from build123d import *

# Parameters (mm, degrees)
BOSS_EXTRUDE1_DEPTH  = 0.762
BOSS_EXTRUDE2_DEPTH  = 2.54
SKETCH4_W            = 6.985
SKETCH4_H            = 4.572
BOSS_EXTRUDE3_DEPTH  = 1.27
FILLET1_R            = 2.54
SKETCH5_W            = 6.985
SKETCH5_H            = 2.032
BOSS_EXTRUDE4_DEPTH  = 0.508
FILLET2_R            = 1.016
FILLET3_R            = 1.016
FILLET2_OF_MIRROR4_R = 1.016
FILLET4_R            = 2.54
FILLET5_R            = 1.016


with BuildPart() as part:
    # Sketch1 → Boss-Extrude1 (new body)
    with BuildSketch(Plane.XY):
        Polygon((-33.378913043, 6.316869565), (16.151086957, 6.316869565), (24.088586957, -1.620630435), (16.151086957, -9.558130435), (-33.378913043, -9.558130435), (-41.316413043, -1.620630435), align=None)
    extrude(amount=BOSS_EXTRUDE1_DEPTH)

    # Sketch2 → Boss-Extrude2 (add)
    with BuildSketch(Plane(origin=(0, 0, 0), x_dir=(-1, 0, 0), z_dir=(0, 0, -1))):
        Polygon((30.521413043, 6.316869565), (33.378913043, 6.316869565), (41.316413043, -1.620630435), (33.378913043, -9.558130435), (30.521413043, -9.558130435), (30.521413043, -8.660104823), (32.480887431, -8.660104823), (39.520361819, -1.620630435), (32.480887431, 5.418843953), (30.521413043, 5.418843953), align=None)
        Polygon((-16.151086957, -9.558130435), (-24.088586957, -1.620630435), (-16.151086957, 6.316869565), (-13.293586957, 6.316869565), (-13.293586957, 5.418843953), (-15.253061344, 5.418843953), (-22.292535732, -1.620630435), (-15.253061344, -8.660104823), (-13.293586957, -8.660104823), (-13.293586957, -9.558130435), align=None)
    extrude(amount=BOSS_EXTRUDE2_DEPTH)

    # Sketch4 → Boss-Extrude3 (add)
    with BuildSketch(Plane(origin=(0, 6.316869565, 0), x_dir=(1, 0, 0), z_dir=(0, 1, 0))):
        with Locations((5.991086957, 1.524)):
            Rectangle(SKETCH4_W, SKETCH4_H)
        with Locations((-23.218913043, 1.524)):
            Rectangle(SKETCH4_W, SKETCH4_H)
    boss_extrude3 = extrude(amount=BOSS_EXTRUDE3_DEPTH)

    # Fillet1
    # the kernel refuses this fillet: 2.54 mm, written as the material it adds along each edge
    with BuildSketch(Plane(origin=(-26.711413043, 6.316869565, 0.762), x_dir=(-1, 0, 0), z_dir=(0, 0, -1)), Plane(origin=(-19.726413043, 6.316869565, 0), x_dir=(1, 0, 0), z_dir=(0, 0, 1)), Plane(origin=(2.498586957, 6.316869565, 0.762), x_dir=(-1, 0, 0), z_dir=(0, 0, -1)), Plane(origin=(9.483586957, 6.316869565, 0), x_dir=(1, 0, 0), z_dir=(0, 0, 1))) as fillet1_piece_1:
        with BuildLine():
            CenterArc((2.199704526, 2.54), FILLET1_R, 210, 60)
            Line((0, 1.27), (0, 0))
            Line((0, 0), (2.199704526, 0))
        make_face()
    extrude(amount=0.762)

    # Sketch5 → Boss-Extrude4 (add)
    with BuildSketch(Plane.XZ.offset(-6.316869565)):
        with Locations((5.991086957, -2.794)):
            Rectangle(SKETCH5_W, SKETCH5_H)
        with Locations((-23.218913043, -2.794)):
            Rectangle(SKETCH5_W, SKETCH5_H)
    boss_extrude4 = extrude(amount=BOSS_EXTRUDE4_DEPTH)

    # Fillet2
    # the kernel refuses this fillet: 1.016 mm, written as the material it takes off along each edge
    with BuildSketch(Plane(origin=(-0.041413043, 5.808869565, -3.81), x_dir=(0, 1, 0), z_dir=(1, 0, 0))) as fillet2_piece_1:
        with BuildLine():
            CenterArc((FILLET2_R, FILLET2_R), FILLET2_R, 180, 90)
            Line((0, FILLET2_R), (-FILLET2_R * 0.02, FILLET2_R))
            Line((-FILLET2_R * 0.02, FILLET2_R), (-FILLET2_R * 0.02, -FILLET2_R * 0.02))
            Line((-FILLET2_R * 0.02, -FILLET2_R * 0.02), (FILLET2_R, -FILLET2_R * 0.02))
            Line((FILLET2_R, -FILLET2_R * 0.02), (FILLET2_R, 0))
        make_face()
    extrude(amount=12.065, mode=Mode.SUBTRACT)
    with BuildSketch(Plane(origin=(11.683291482, 5.808869565, -1.778), x_dir=(0, 0, -1), z_dir=(-1, 0, 0))) as fillet2_piece_2:
        with BuildLine():
            CenterArc((0.87988181, -1.016), FILLET2_R, 90, 60)
            Line((0, -0.508), (-0.017597636, -0.49784))
            ThreePointArc((-0.017597636, -0.49784), (-0.02032, -0.254), (-0.02032, 0))
            Line((-0.02032, 0), (0, 0.02032))
            Line((0, 0.02032), (0.87988181, 0.02032))
            Line((0.87988181, 0.02032), (0.87988181, 0))
        make_face()
    extrude(amount=11.384409051, mode=Mode.SUBTRACT)
    with BuildSketch(Plane(origin=(-29.251413043, 5.808869565, -3.81), x_dir=(0, 0, 1), z_dir=(1, 0, 0))) as fillet2_piece_3:
        with BuildLine():
            CenterArc((FILLET2_R, -FILLET2_R), FILLET2_R, 90, 90)
            Line((0, -FILLET2_R), (-FILLET2_R * 0.02, -FILLET2_R))
            Line((-FILLET2_R * 0.02, -FILLET2_R), (-FILLET2_R * 0.02, FILLET2_R * 0.02))
            Line((-FILLET2_R * 0.02, FILLET2_R * 0.02), (FILLET2_R, FILLET2_R * 0.02))
            Line((FILLET2_R, FILLET2_R * 0.02), (FILLET2_R, 0))
        make_face()
    extrude(amount=12.065, mode=Mode.SUBTRACT)
    with BuildSketch(Plane(origin=(-17.526708518, 5.808869565, -1.778), x_dir=(0, 1, 0), z_dir=(-1, 0, 0))) as fillet2_piece_4:
        with BuildLine():
            CenterArc((1.016, 0.87988181), FILLET2_R, 180, 60)
            Line((0, 0.87988181), (-0.02032, 0.87988181))
            Line((-0.02032, 0.87988181), (-0.02032, 0))
            Line((-0.02032, 0), (0, -0.02032))
            ThreePointArc((0, -0.02032), (0.254, -0.02032), (0.49784, -0.017597636))
            Line((0.49784, -0.017597636), (0.508, 0))
        make_face()
    extrude(amount=11.384409051, mode=Mode.SUBTRACT)

    # Fillet3
    # the kernel refuses this fillet: 1.016 mm, written as the material it adds along each edge
    with BuildSketch(Plane(origin=(-26.711413043, 10.126869565, 0), x_dir=(-1, 0, 0), z_dir=(0, -1, 0))) as fillet3_piece_1_section:
        with BuildLine():
            CenterArc((FILLET3_R, FILLET3_R), FILLET3_R, 180, 90)
            Line((0, FILLET3_R), (0, 0))
            Line((0, 0), (FILLET3_R, 0))
        make_face()
    fillet3_piece_1 = extrude(amount=3.81, mode=Mode.PRIVATE)
    fillet3_piece_1 = fillet3_piece_1 - Plane(origin=(-28.911117569, 8.856869565, 0), x_dir=(-1, 0, 0), z_dir=(0, 0, 1)) * Cylinder(2.54, 12, mode=Mode.PRIVATE)
    add(fillet3_piece_1)
    with BuildSketch(Plane(origin=(-19.726413043, 10.126869565, 0), x_dir=(1, 0, 0), z_dir=(0, -1, 0))) as fillet3_piece_2_section:
        with BuildLine():
            CenterArc((FILLET3_R, -FILLET3_R), FILLET3_R, 90, 90)
            Line((0, -FILLET3_R), (0, 0))
            Line((0, 0), (FILLET3_R, 0))
        make_face()
    fillet3_piece_2 = extrude(amount=3.81, mode=Mode.PRIVATE)
    fillet3_piece_2 = fillet3_piece_2 - Plane(origin=(-17.526708518, 8.856869565, 0), x_dir=(1, 0, 0), z_dir=(0, 0, -1)) * Cylinder(2.54, 12, mode=Mode.PRIVATE)
    add(fillet3_piece_2)
    with BuildSketch(Plane(origin=(2.498586957, 10.126869565, 0), x_dir=(-1, 0, 0), z_dir=(0, -1, 0))) as fillet3_piece_3_section:
        with BuildLine():
            CenterArc((FILLET3_R, FILLET3_R), FILLET3_R, 180, 90)
            Line((0, FILLET3_R), (0, 0))
            Line((0, 0), (FILLET3_R, 0))
        make_face()
    fillet3_piece_3 = extrude(amount=3.81, mode=Mode.PRIVATE)
    fillet3_piece_3 = fillet3_piece_3 - Plane(origin=(0.298882431, 8.856869565, 0), x_dir=(-1, 0, 0), z_dir=(0, 0, 1)) * Cylinder(2.54, 12, mode=Mode.PRIVATE)
    add(fillet3_piece_3)
    with BuildSketch(Plane(origin=(9.483586957, 10.126869565, 0), x_dir=(1, 0, 0), z_dir=(0, -1, 0))) as fillet3_piece_4_section:
        with BuildLine():
            CenterArc((FILLET3_R, -FILLET3_R), FILLET3_R, 90, 90)
            Line((0, -FILLET3_R), (0, 0))
            Line((0, 0), (FILLET3_R, 0))
        make_face()
    fillet3_piece_4 = extrude(amount=3.81, mode=Mode.PRIVATE)
    fillet3_piece_4 = fillet3_piece_4 - Plane(origin=(11.683291482, 8.856869565, 0), x_dir=(1, 0, 0), z_dir=(0, 0, -1)) * Cylinder(2.54, 12, mode=Mode.PRIVATE)
    add(fillet3_piece_4)

    # Mirror4: Boss-Extrude3, Boss-Extrude4 across plane
    add(boss_extrude3.mirror(Plane.ZX.offset(-1.620630435)))
    add(boss_extrude4.mirror(Plane.ZX.offset(-1.620630435)))

    # Fillet2 of Mirror4
    # the kernel refuses this fillet: 1.016 mm, written as the material it takes off along each edge
    with BuildSketch(Plane(origin=(-0.041413043, -9.050130435, -3.81), x_dir=(0, 0, 1), z_dir=(1, 0, 0)), Plane(origin=(-29.251413043, -9.050130435, -3.81), x_dir=(0, 0, 1), z_dir=(1, 0, 0))) as fillet2_of_mirror4_piece_1:
        with BuildLine():
            CenterArc((FILLET2_OF_MIRROR4_R, FILLET2_OF_MIRROR4_R), FILLET2_OF_MIRROR4_R, 180, 90)
            Line((0, FILLET2_OF_MIRROR4_R), (-FILLET2_OF_MIRROR4_R * 0.02, FILLET2_OF_MIRROR4_R))
            Line((-FILLET2_OF_MIRROR4_R * 0.02, FILLET2_OF_MIRROR4_R), (-FILLET2_OF_MIRROR4_R * 0.02, -FILLET2_OF_MIRROR4_R * 0.02))
            Line((-FILLET2_OF_MIRROR4_R * 0.02, -FILLET2_OF_MIRROR4_R * 0.02), (FILLET2_OF_MIRROR4_R, -FILLET2_OF_MIRROR4_R * 0.02))
            Line((FILLET2_OF_MIRROR4_R, -FILLET2_OF_MIRROR4_R * 0.02), (FILLET2_OF_MIRROR4_R, 0))
        make_face()
    extrude(amount=12.065, mode=Mode.SUBTRACT)
    with BuildSketch(Plane(origin=(11.683291482, -9.050130435, -1.778), x_dir=(0, 0, -1), z_dir=(-1, 0, 0)), Plane(origin=(-17.526708518, -9.050130435, -1.778), x_dir=(0, 0, -1), z_dir=(-1, 0, 0))) as fillet2_of_mirror4_piece_2:
        with BuildLine():
            CenterArc((0.87988181, 1.016), FILLET2_OF_MIRROR4_R, 210, 60)
            Line((0, 0.508), (-0.017597636, 0.49784))
            ThreePointArc((-0.017597636, 0.49784), (-0.02032, 0.254), (-0.02032, 0))
            Line((-0.02032, 0), (0, -0.02032))
            Line((0, -0.02032), (0.87988181, -0.02032))
            Line((0.87988181, -0.02032), (0.87988181, 0))
        make_face()
    extrude(amount=11.384409051, mode=Mode.SUBTRACT)

    # Fillet4
    # the kernel refuses this fillet: 2.54 mm, written as the material it adds along each edge
    with BuildSketch(Plane(origin=(-26.711413043, -9.558130435, 0.762), x_dir=(-1, 0, 0), z_dir=(0, 0, -1)), Plane(origin=(-19.726413043, -9.558130435, 0), x_dir=(1, 0, 0), z_dir=(0, 0, 1)), Plane(origin=(2.498586957, -9.558130435, 0.762), x_dir=(-1, 0, 0), z_dir=(0, 0, -1)), Plane(origin=(9.483586957, -9.558130435, 0), x_dir=(1, 0, 0), z_dir=(0, 0, 1))) as fillet4_piece_1:
        with BuildLine():
            CenterArc((2.199704526, -2.54), FILLET4_R, 90, 60)
            Line((0, -1.27), (0, 0))
            Line((0, 0), (2.199704526, 0))
        make_face()
    extrude(amount=0.762)

    # Fillet5
    # the kernel refuses this fillet: 1.016 mm, written as the material it adds along each edge
    with BuildSketch(Plane(origin=(-26.711413043, -13.368130435, 0), x_dir=(-1, 0, 0), z_dir=(0, 1, 0))) as fillet5_piece_1_section:
        with BuildLine():
            CenterArc((FILLET5_R, -FILLET5_R), FILLET5_R, 90, 90)
            Line((0, -FILLET5_R), (0, 0))
            Line((0, 0), (FILLET5_R, 0))
        make_face()
    fillet5_piece_1 = extrude(amount=3.81, mode=Mode.PRIVATE)
    fillet5_piece_1 = fillet5_piece_1 - Plane(origin=(-28.911117569, -12.098130435, 0), x_dir=(-1, 0, 0), z_dir=(0, 0, 1)) * Cylinder(2.54, 12, mode=Mode.PRIVATE)
    add(fillet5_piece_1)
    with BuildSketch(Plane(origin=(9.483586957, -13.368130435, 0), x_dir=(1, 0, 0), z_dir=(0, 1, 0))) as fillet5_piece_2_section:
        with BuildLine():
            CenterArc((FILLET5_R, FILLET5_R), FILLET5_R, 180, 90)
            Line((0, FILLET5_R), (0, 0))
            Line((0, 0), (FILLET5_R, 0))
        make_face()
    fillet5_piece_2 = extrude(amount=3.81, mode=Mode.PRIVATE)
    fillet5_piece_2 = fillet5_piece_2 - Plane(origin=(11.683291482, -12.098130435, 0), x_dir=(1, 0, 0), z_dir=(0, 0, -1)) * Cylinder(2.54, 12, mode=Mode.PRIVATE)
    add(fillet5_piece_2)
    with BuildSketch(Plane(origin=(-19.726413043, -13.368130435, 0), x_dir=(1, 0, 0), z_dir=(0, 1, 0))) as fillet5_piece_3_section:
        with BuildLine():
            CenterArc((FILLET5_R, FILLET5_R), FILLET5_R, 180, 90)
            Line((0, FILLET5_R), (0, 0))
            Line((0, 0), (FILLET5_R, 0))
        make_face()
    fillet5_piece_3 = extrude(amount=3.81, mode=Mode.PRIVATE)
    fillet5_piece_3 = fillet5_piece_3 - Plane(origin=(-17.526708518, -12.098130435, 0), x_dir=(1, 0, 0), z_dir=(0, 0, -1)) * Cylinder(2.54, 12, mode=Mode.PRIVATE)
    add(fillet5_piece_3)
    with BuildSketch(Plane(origin=(2.498586957, -13.368130435, 0), x_dir=(-1, 0, 0), z_dir=(0, 1, 0))) as fillet5_piece_4_section:
        with BuildLine():
            CenterArc((FILLET5_R, -FILLET5_R), FILLET5_R, 90, 90)
            Line((0, -FILLET5_R), (0, 0))
            Line((0, 0), (FILLET5_R, 0))
        make_face()
    fillet5_piece_4 = extrude(amount=3.81, mode=Mode.PRIVATE)
    fillet5_piece_4 = fillet5_piece_4 - Plane(origin=(0.298882431, -12.098130435, 0), x_dir=(-1, 0, 0), z_dir=(0, 0, 1)) * Cylinder(2.54, 12, mode=Mode.PRIVATE)
    add(fillet5_piece_4)


solid = part.part
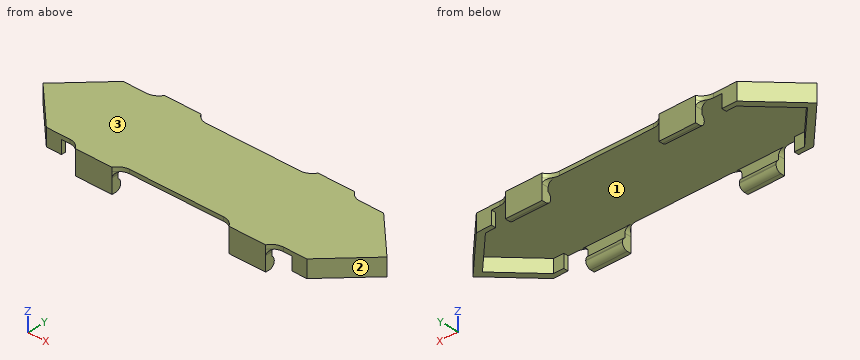
CAD build for the part. Positions are in the model's coordinates, mm. Face numbers are marked on the shaded views. Give positions to 0.01 mm unless a question says otherwise; leave off trailing zeros. Loops run counter-clockwise (first coordinate to the right, second up) from the corner with the lowest first, then second, coordinate; pieces in that order, holes last. Notation, with made-up numbers: M 48.5,-31 L 83.5,-31 A31 cw 83.5,5 Z; hole C 15,13 d9. An arc over 180 degrees is marked long. Answer in a Markdown table with one row per item. Add a question column.
Item 1: Probe probe 1 along Y at (x, z) = (3, -1.1); probe 2 along Y at (x, z) = (14.5, 0.1); probe 3 along Z at (x, y) = (-13, -3.75). List the from-to ranges inside material, lowest first.
Item 2: Drop flat-ended pins along their axis: P1, Ø1.5, axis at y = -3.5, z = -2.5, coming from the +X side; P2, Ø2, axis at y = -10, z = -2.5, coming from the -X side; P3, Ø0.5, axis at y = -10, z = -2.5, coming from the +X side. Give the stop position or say it passes through.
Item 3: Band-saw the part on A-A on x = -22. Give the cut face in (y, z), then the cut area to 3 significant figures.
Item 4: Mould opens along X. For the marked faces 1, 2 and 3 say: +X half, -X half, draft (parallel to the pull), parting line (faces both ways), or undercut.
Item 5: Band-saw the part on B-B on y = 3. Give the cut face in (x, z), then the cut area to 3 significant figures.
Item 6: Band-saw the part on D-D on x = -2. Give the cut face in (y, z).
Item 7: Band-saw the part on C-C on x = 20. Give the cut face in (y, z), then the cut area to 3 significant figures.
Reply:
| question | item | result |
|---|---|---|
| 1 | probe 1 | y = -10.83 to -9.56, 6.32 to 7.59 |
| 1 | probe 2 | y = -9.56 to 6.32 |
| 1 | probe 3 | z = 0 to 0.76 |
| 2 | P1 | stops at x = 22.96 |
| 2 | P2 | stops at x = -33.94 |
| 2 | P3 | stops at x = 9.48 |
| 3 | outline | M -10.83,-3.81 L -10.07,-3.81 A1.02 ccw -9.05,-2.79 L -9.05,-2.66 A1.02 ccw -9.56,-1.78 L -9.56,0 L 6.32,0 L 6.32,-1.78 A1.02 ccw 5.81,-2.66 L 5.81,-2.79 A1.02 ccw 6.82,-3.81 L 7.59,-3.81 L 7.59,0.76 L -10.83,0.76 Z |
| 3 | area | 25.1 mm^2 |
| 4 | face 1 | undercut |
| 4 | face 2 | +X half |
| 4 | face 3 | draft |
| 5 | outline | M -36.7,-2.54 L -34.9,-2.54 L -34.9,0 L 17.67,0 L 17.67,-2.54 L 19.47,-2.54 L 19.47,0.76 L -36.7,0.76 Z |
| 5 | area | 51.9 mm^2 |
| 6 | outline | M -9.56,0 L 6.32,0 L 6.32,0.76 L -9.56,0.76 Z |
| 7 | outline | M -5.71,-2.54 L -3.91,-2.54 L -3.91,0 L 0.67,0 L 0.67,-2.54 L 2.47,-2.54 L 2.47,0.76 L -5.71,0.76 Z |
| 7 | area | 15.4 mm^2 |
